from build123d import *

# Parameters (mm, degrees)
BOSS_EXTRUDE1_DEPTH = 3.175
BOSS_EXTRUDE2_DEPTH = 25.4
SKETCH4_R           = 3.175
BOSS_EXTRUDE3_DEPTH = 23.876
SKETCH5_W           = 65
SKETCH5_H           = 35.5
BOSS_EXTRUDE4_DEPTH = 21.14


with BuildPart() as part:
    # Sketch1 → Boss-Extrude1 (new body)
    with BuildSketch(Plane(origin=(0, 0, 0), x_dir=(1, 0, 0), z_dir=(0, 1, 0))):
        with BuildLine():
            Line((0, 0), (-107.95, 0))
            add(Edge.make_bspline(
                [(-107.95, 0), (-111.264371581, -22.223355165), (-93.128309356, -45.976040953), (-57.609622492, -57.69778745), (-28.725306534, -52.845882242), (-11.819511833, -42.209688066), (0, -44.45)],
                knots=[0, 0, 0, 0, 0.396763779, 0.585186104, 0.766934878, 1, 1, 1, 1], degree=3))
            Line((0, -44.45), (0, 0))
        make_face()
    extrude(amount=BOSS_EXTRUDE1_DEPTH)

    # Sketch3 → Boss-Extrude2 (add)
    with BuildSketch(Plane(origin=(0, 3.175, 0), x_dir=(1, 0, 0), z_dir=(0, 1, 0))):
        with BuildLine():
            Line((-107.95, 0), (0, 0))
            Line((0, 0), (0, -44.45))
            add(Edge.make_bspline(
                [(-107.95, 0), (-111.264371581, -22.223355165), (-93.128309356, -45.976040953), (-57.609622492, -57.69778745), (-28.725306534, -52.845882242), (-11.819511833, -42.209688066), (0, -44.45)],
                knots=[0, 0, 0, 0, 0.396763779, 0.585186104, 0.766934878, 1, 1, 1, 1], degree=3))
        make_face()
        with BuildLine():
            Line((-3.175, -3.175), (-3.175, -40.851813342))
            add(Edge.make_bspline(
                [(-3.175, -40.851813342), (-3.981241555, -40.799236826), (-5.613173677, -40.758071121), (-8.755907484, -40.91833994), (-12.544966377, -41.515078302), (-16.858992044, -42.692888995), (-22.365050245, -44.656719953), (-27.607498849, -46.904281185), (-32.742546929, -48.882210607), (-37.923615998, -50.544033975), (-44.576686254, -52.030970183), (-52.639871626, -52.729404253), (-60.625408491, -52.20082035), (-68.513307445, -50.421711202), (-76.136701649, -47.534738566), (-83.353587797, -43.660935754), (-89.925307122, -38.936837432), (-95.60948708, -33.390844892), (-100.196904726, -27.060690394), (-102.946013069, -21.145493232), (-104.40794392, -16.016511773), (-105.110198278, -11.965850914), (-105.342998437, -8.407656976), (-105.303439388, -5.46128014), (-105.203482374, -3.930833291), (-105.134910032, -3.175)],
                knots=[0.017398094, 0.017398094, 0.017398094, 0.017398094, 0.032397512, 0.047396929, 0.077395765, 0.107394601, 0.137393436, 0.197391108, 0.227389943, 0.257388779, 0.31738645, 0.377384122, 0.437381793, 0.497379464, 0.557377136, 0.617374807, 0.677372478, 0.73737015, 0.797367821, 0.857365492, 0.887364328, 0.917363164, 0.947361999, 0.962361417, 0.977360835, 0.977360835, 0.977360835, 0.977360835], degree=3))
            Line((-105.134910032, -3.175), (-3.175, -3.175))
        make_face(mode=Mode.SUBTRACT)
    extrude(amount=-BOSS_EXTRUDE2_DEPTH)

    # Sketch4 → Boss-Extrude3 (add)
    with BuildSketch(Plane(origin=(0, -22.225, 0), x_dir=(-1, 0, 0), z_dir=(0, -1, 0))):
        with Locations((105.134910032, -3.175)):
            Circle(SKETCH4_R)
        with Locations((3.175, -3.175)):
            Circle(SKETCH4_R)
        with Locations((3.175, -40.851813342)):
            Circle(SKETCH4_R)
    extrude(amount=-BOSS_EXTRUDE3_DEPTH)

    # Sketch5 → Boss-Extrude4 (add)
    with BuildSketch(Plane.XZ):
        with Locations((-38.85, 20.925)):
            Rectangle(SKETCH5_W, SKETCH5_H)
    extrude(amount=BOSS_EXTRUDE4_DEPTH)


solid = part.part
Check sheet for the modelled part. Datum: model origin and axes. Units: mm. A direction names the side the tool comes from. Round coordinates to 2 decimals unless told otherwise and drop trailing zeros. Return JSON: item names as keys, results as strings.
Q1. Draft check along X on faces 3 (the flat face through (-39, -10, 38.675)), 4 (the flat face through (0, -9, 22)), 5 (the flat face through (-55, -9, 0)). Enter one of: released by +X, released by -X, zero draft, split by the parting line, or undercut.
Returned:
{"face 3": "undercut", "face 4": "released by +X", "face 5": "zero draft"}
Q2. Access from +Z, -Z, +X, -X, +Y, -Y to the whole of each face (thin tool, end or side, straight path). Record for faces 1 (the flat face through (-71.35, -10, 21)), 2 (the flat face through (-56, 3.175, 22)).
Returned:
{"face 1": "-Y", "face 2": "+Z, -Z, +X, -X, +Y"}
Q3. Depth check by flat-ended pin: P1, Ø10, axis at x = -93.5, y = -14.5, coming from the +Z side; P2, Ø5, axis at y = -2, z = 44, coming from the -X side; P3, Ø8, axis at x = -66, y = 0.5, coming from the +Z side. Enter the tip coordinate at first touch or a pass-through.
Returned:
{"P1": "stops at z = 43.81", "P2": "stops at x = -91.5", "P3": "stops at z = 54.99"}
Q4. Scan lines: L1, parallel to X at y = -8.25, z = 7.5 (3 decimals); L2, parallel to X at y = -20, z = 20.5 (3 decimals); L3, parallel to Z at x = -18, y = -12.75 (3 decimals). Record each from-to range of solid material in increasing order. Write a range as from..to.
Returned:
{"L1": "x = -108.491..-105.316, -71.35..-6.35, -3.175..0", "L2": "x = -106.375..-103.014, -71.35..-6.35, -3.175..0", "L3": "z = 0..38.675, 43.123..46.482"}
